Input: part model. Units: mm. Frame: model coordinates. Face numbers are marked on the shaded views. Give positions to 0.01 mm unless a question says otherwise; leave off trailing zeros. Order: outer loops, then holes, each group sorted by start corner. A loop starts at its lowest first (then second) coordinate and runs counter-clockwise, first axis right, second up. Notation, with made-up numbers: (46, 31) - (50, 31) arc R19 ccw to (50, 51) - close; hole circle Ø3 at (77, 18). An arc over 180 degrees is marked (long way). Use a Markdown table: item, result.
from build123d import *

# Parameters (mm, degrees)
SKETCH_1_W             = 98
SKETCH_1_H             = 108
EXTRUDE_1_DEPTH        = 4
SKETCH_2_R             = 11.5
CUT_EXTRUDE_1_DEPTH    = 10
SKETCH_3_R             = 32.6
CUT_EXTRUDE_2_DEPTH    = 3
SKETCH_4_R             = 1.5
CUT_EXTRUDE_3_DEPTH    = 2
FILLET_1_R             = 5
HOLE_WIZARD_M4_1_D     = 3.3
HOLE_WIZARD_M4_1_DEPTH = 10.1
HOLE_WIZARD_M4_1_TIP   = 0.991420021
HOLE_WIZARD_M3_1_D     = 2.5
HOLE_WIZARD_M3_1_DEPTH = 7.5
HOLE_WIZARD_M3_1_TIP   = 0.751075774
HOLE_WIZARD_M3_2_D     = 2.5
HOLE_WIZARD_M3_2_DEPTH = 7.5
HOLE_WIZARD_M3_2_TIP   = 0.751075774


with BuildPart() as part:
    # 草图1 → 凸台-拉伸1 (new body)
    with BuildSketch(Plane.XY):
        Rectangle(SKETCH_1_W, SKETCH_1_H)
    extrude(amount=EXTRUDE_1_DEPTH)

    # 草图2 → 切除-拉伸1 (cut)
    with BuildSketch(Plane.XY.offset(4)):
        Circle(SKETCH_2_R)
    extrude(amount=-CUT_EXTRUDE_1_DEPTH, mode=Mode.SUBTRACT)

    # 草图3 → 切除-拉伸2 (cut)
    with BuildSketch(Plane.XY.offset(4)):
        Circle(SKETCH_3_R)
    extrude(amount=-CUT_EXTRUDE_2_DEPTH, mode=Mode.SUBTRACT)

    # 草图4 → 切除-拉伸3 (cut)
    with BuildSketch(Plane.XY.offset(1)):
        with Locations((-10.606601718, 10.606601718)):
            Circle(SKETCH_4_R)
        with Locations((10.606601718, -10.606601718)):
            Circle(SKETCH_4_R)
        with Locations((10.606601718, 10.606601718)):
            Circle(SKETCH_4_R)
        with Locations((-10.606601718, -10.606601718)):
            Circle(SKETCH_4_R)
    extrude(amount=-CUT_EXTRUDE_3_DEPTH, mode=Mode.SUBTRACT)

    # 圆角1
    fillet_1_edges = [part.edges().sort_by_distance(p)[0] for p in [
        (-49, 54, 2),
        (49, 54, 2),
        (49, -54, 2),
        (-49, -54, 2),
    ]]
    fillet(fillet_1_edges, radius=FILLET_1_R)

    # M4 螺纹孔1
    with Locations(Plane(origin=(0, 0, 0), x_dir=(-1, 0, 0), z_dir=(0, 0, -1))):
        with Locations((-25, 49), (-25, 34), (25, 34), (25, 49), (-25, -34), (-25, -49), (25, -49), (25, -34)):
            Hole(HOLE_WIZARD_M4_1_D / 2, depth=HOLE_WIZARD_M4_1_DEPTH)
            with Locations((0, 0, -(HOLE_WIZARD_M4_1_DEPTH + HOLE_WIZARD_M4_1_TIP / 2))):  # 118° drill point
                Cone(0, HOLE_WIZARD_M4_1_D / 2, HOLE_WIZARD_M4_1_TIP, mode=Mode.SUBTRACT)

    # M3 螺纹孔1
    with Locations(Plane(origin=(0, 0, 0), x_dir=(-1, 0, 0), z_dir=(0, 0, -1))):
        with Locations((41, 2), (34, 11)):
            Hole(HOLE_WIZARD_M3_1_D / 2, depth=HOLE_WIZARD_M3_1_DEPTH)
            with Locations((0, 0, -(HOLE_WIZARD_M3_1_DEPTH + HOLE_WIZARD_M3_1_TIP / 2))):  # 118° drill point
                Cone(0, HOLE_WIZARD_M3_1_D / 2, HOLE_WIZARD_M3_1_TIP, mode=Mode.SUBTRACT)

    # M3 螺纹孔2
    with Locations(Plane.XY.offset(4)):
        with Locations((38.97114317, 22.5), (45, 0), (38.97114317, -22.5)):
            Hole(HOLE_WIZARD_M3_2_D / 2, depth=HOLE_WIZARD_M3_2_DEPTH)
            with Locations((0, 0, -(HOLE_WIZARD_M3_2_DEPTH + HOLE_WIZARD_M3_2_TIP / 2))):  # 118° drill point
                Cone(0, HOLE_WIZARD_M3_2_D / 2, HOLE_WIZARD_M3_2_TIP, mode=Mode.SUBTRACT)


solid = part.part
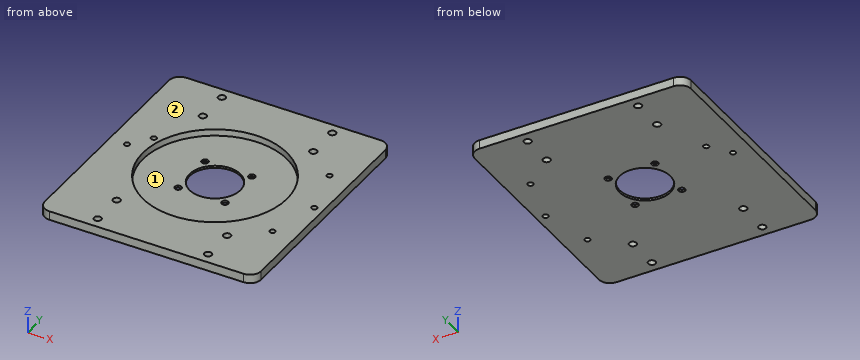
1. Section query D-D (y = -3). Return loops of the section in (x, z), then the cut area to 3 significant figures.
Response:
| item | result |
|---|---|
| outline | (-49, 0) - (-11.1, 0) - (-11.1, 1) - (-32.46, 1) - (-32.46, 4) - (-49, 4) - close; (11.1, 0) - (49, 0) - (49, 4) - (32.46, 4) - (32.46, 1) - (11.1, 1) - close |
| area | 175 mm^2 |
2. Material intervals for line 1 along Z through (x, y) = (-30, -3); line 2 along Y through (x, z) = (-11.5, 3.3); line 3 along Y through (x, z) = (-17.5, 1.3), sorted ascending.
Response:
| item | result |
|---|---|
| line 1 | z = 0 to 1 |
| line 2 | y = -54 to -30.5, 30.5 to 54 |
| line 3 | y = -54 to -27.5, 27.5 to 54 |
3. Mould query, pull axis X, two halves, no side actions, for the marked faces 1 and 2. Classes: pulls with the +X half, pulls with the -X half, needs draft (parallel to the pull), parting line crosses it, or undercut.
Response:
| item | result |
|---|---|
| face 1 | undercut |
| face 2 | needs draft |
4. Pin query (flat end, axial travel): pin 1 (10 mm diameter, centred on x = 5, y = 11.5, fed in from +Z); pin 2 (1.8 mm diameter, centred on x = -10.61, y = 10.61, fed in from -Z). Return the tip coordinate at first contact, or that it passes through.
Response:
| item | result |
|---|---|
| pin 1 | stops at z = 1 |
| pin 2 | passes through |
5. Section query C-C (x = -34). Return loops of the section in (y, z).
Response:
| item | result |
|---|---|
| outline | (-54, 0) - (9.75, 0) - (9.75, 4) - (-54, 4) - close; (12.25, 0) - (54, 0) - (54, 4) - (12.25, 4) - close |
6. Section query A-A (y = 34). Return loops of the section in (x, z).
Response:
| item | result |
|---|---|
| outline | (-49, 0) - (-26.65, 0) - (-26.65, 4) - (-49, 4) - close; (-23.35, 0) - (23.35, 0) - (23.35, 4) - (-23.35, 4) - close; (26.65, 0) - (49, 0) - (49, 4) - (26.65, 4) - close |
7. Section query B-B (z = 3.25). State how many separate pieces and enclosed holes the cut face has, then the cut area to 3 significant figures.
Response:
| item | result |
|---|---|
| separate pieces | 1 |
| enclosed holes | 14 |
| area | 7,130 mm^2 |
